CAD build for the part. Positions are in the model's coordinates, mm. A direction names the side the tool comes from. Round coordinates to 2 decimals unless told otherwise and drop trailing zeros. Order: outer loops, then holes, each group sorted by start corner. A loop starts at its lowest first (then second) coordinate and runs counter-clockwise, first axis right, second up. Notation, with made-up numbers: M -13,62.25 L 26,62.25 A11 ccw 26,75.25 Z; hole C 54,22.5 d8. An arc over 180 degrees is marked long. Put each result on its own line as item: value.
```python
from build123d import *

# Parameters (mm, degrees)
SKETCH_W     = 63.8
SKETCH_H     = 16.2
PAD_DEPTH    = 7
THICKNESS_T  = -2
SKETCH001_W  = 1.4
SKETCH001_H  = 1.4
PAD001_DEPTH = 5


with BuildPart() as part:
    # Sketch → Pad (new body)
    with BuildSketch(Plane.XY):
        with Locations((31.9, 8.1)):
            Rectangle(SKETCH_W, SKETCH_H)
    extrude(amount=PAD_DEPTH)

    # Thickness
    thickness_openings = [part.faces().sort_by_distance(p)[0] for p in [
        (31.9, 8.1, 7),
        (63.8, 8.1, 3.5),
        (0, 8.1, 3.5),
    ]]
    offset(amount=THICKNESS_T, openings=thickness_openings)

    # Sketch001 (on Face10 of Thickness) → Pad001 (join)
    with BuildSketch(Plane.XY.offset(2)):
        with Locations((31.9, 13.5)):
            Rectangle(SKETCH001_W, SKETCH001_H)
        with Locations((31.9, 2.7)):
            Rectangle(SKETCH001_W, SKETCH001_H)
    extrude(amount=PAD001_DEPTH)


solid = part.part
```
Item 1: Band-saw the part on C-C on y = 4.25. Give the cut face in (x, z).
Answers below:
outline: M 0,0 L 63.8,0 L 63.8,2 L 0,2 Z
Item 2: Probe line 1 along Y through (x, z) = (12.5, 5.25); line 2 along Z through (x, y) = (21, 7); line 3 along X through (y, z) = (2.5, 2.5). List the from-to ranges inside material, lowest first. Write a range as [from, to].
Answers below:
line 1: [0, 2], [14.2, 16.2]
line 2: [0, 2]
line 3: [31.2, 32.6]
Item 3: Band-saw the part on B-B on x = 35. Give the cut face in (y, z), and give its area (3 significant figures).
Answers below:
outline: M 0,0 L 16.2,0 L 16.2,7 L 14.2,7 L 14.2,2 L 2,2 L 2,7 L 0,7 Z
area: 52.4 mm²
Item 4: Mould opens along Y. For faces 1 (the flat face through (31, 16.2, 3)), 2 (the flat face through (31, 1, 7)), 3 (the flat face through (31.2, 13, 4)), 4 (the flat face through (32, 3.4, 4)) say: pulls with the +Y half, pulls with the -Y half, needs draft (parallel to the pull), parting line crosses it, or undercut.
Answers below:
face 1: pulls with the +Y half
face 2: needs draft
face 3: undercut
face 4: undercut
Item 5: Band-saw the part on A-A on z = 3.5. Give the cut face in (x, y), and give its area (3 significant figures).
Answers below:
outline: M 0,0 L 63.8,0 L 63.8,2 L 32.6,2 L 32.6,3.4 L 31.2,3.4 L 31.2,2 L 0,2 Z; M 0,14.2 L 31.2,14.2 L 31.2,12.8 L 32.6,12.8 L 32.6,14.2 L 63.8,14.2 L 63.8,16.2 L 0,16.2 Z
area: 259 mm²
Item 6: Pin check, flat tip, straight feed: P1, Ø1.1, axis at y = 3, z = 5, coming from the -X side. Stop position of the tip, or through.
Answers below:
P1: x = 31.2
Item 7: Tool access for faces 5 (the flat face through (32, 12.8, 4)), 6 (the flat face through (48, 14.2, 4)), 7 (the flat face through (15, 14.2, 4)): list every direction of +Z, -Z, +X, -X, +Y, -Y with a clear straight run to the whole face (end or side of a thin tool).
Answers below:
face 5: +Z, +X, -X
face 6: +Z, +X
face 7: +Z, -X
